Can you work these out from the drawing? Everything is in mm from the part's minimum corner. A direction names the side the tool comes from. Round coordinates to 2 decimals unless told otherwise and drop trailing zeros. Write each loop counter-clockwise with the first axis right and the second up, starting at its lowest first coordinate (ties: lowest second). Pieces come first, ordered by that corner, then holes. Notation, with made-up numbers: (-2, 53) -> (18, 53) arc R12 ccw to (18, 76) -> close; hole circle Ø2 at (42, 48). An arc over 180 degrees is marked (long way). Put each result on its own line as item: value. Start each with the question number.
1. Suppose I cut it at A-A (y = 6). Please give me the cut outline in (x, z).
2. For pin 1 (3 mm diameter, centred on x = 8, y = 10.5, fed in from +Z); pin 2 (1 mm diameter, centred on y = 4, z = 19, fed in from -X); pin 3 (2 mm diameter, centred on x = 18, z = 6.5, fed in from -Y); pin 4 (1.5 mm diameter, centred on x = 29.5, y = 8.5, fed in from +Z), each with a flat end and sliding along its axis, tell me the tip position at first contact or that it passes through.
3. Suppose I cut it at D-D (z = 19). Please give me the cut outline in (x, y).
4. Which directions (+Z, -Z, +X, -X, +Y, -Y) give clear straight access to the entire face, cutting with the end or side of a thin tool? Please do the marked faces 1, 2, 3, 4 and 5.
5. I need wall thicknesses on probe 1 along Y at (x, z) = (2.25, 16.85); probe 2 along Z at (x, y) = (20, 7.75); probe 3 along X at (y, z) = (7, 3.75). Which ranges of each line are inside material? Lowest first, please. Write a range as from..to.
6. Suppose I cut it at C-C (y = 8.5). Please give me the cut outline in (x, z).
7. Suppose I cut it at B-B (x = 2.25). Please give me the cut outline in (y, z), then the cut area to 3 significant figures.
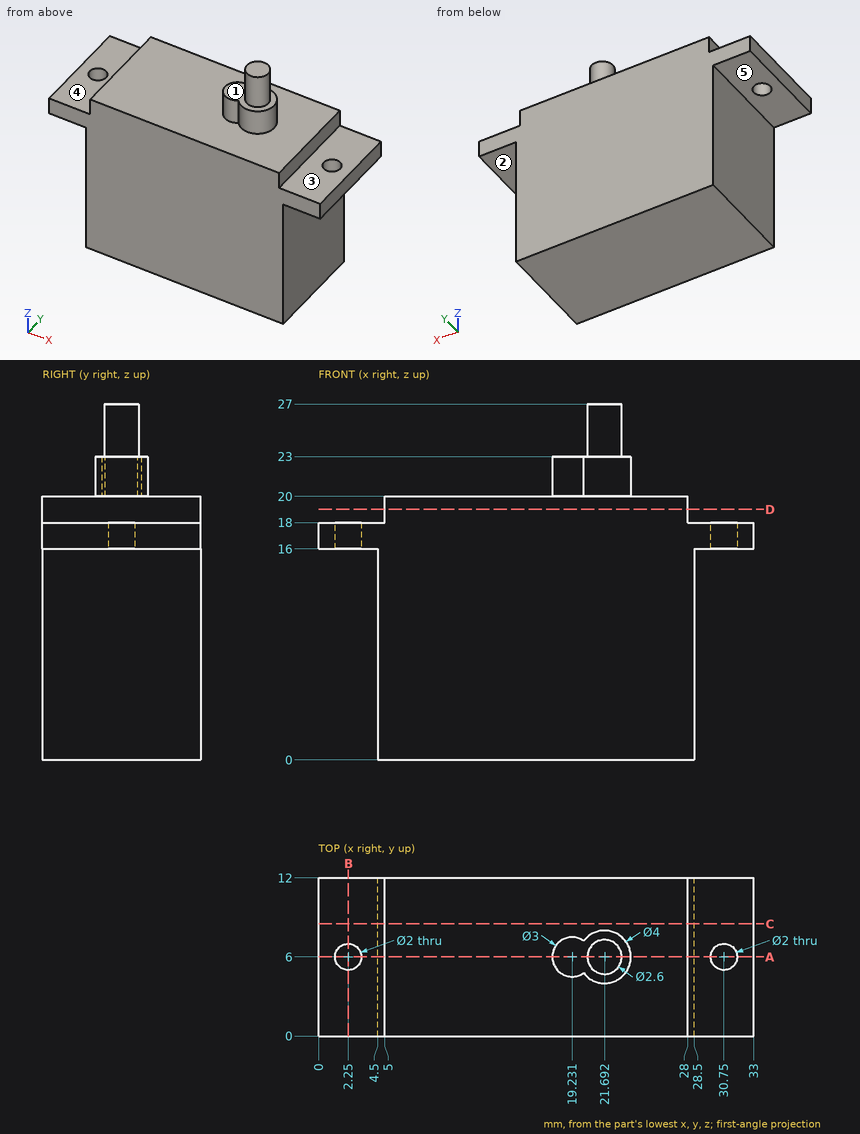
Verdict:
1. outline: (0, 16) -> (1.25, 16) -> (1.25, 18) -> (0, 18) -> close; (3.25, 16) -> (4.5, 16) -> (4.5, 0) -> (28.5, 0) -> (28.5, 16) -> (29.75, 16) -> (29.75, 18) -> (28, 18) -> (28, 20) -> (23.69, 20) -> (23.69, 23) -> (22.99, 23) -> (22.99, 27) -> (20.39, 27) -> (20.39, 23) -> (17.73, 23) -> (17.73, 20) -> (5, 20) -> (5, 18) -> (3.25, 18) -> close; (31.75, 16) -> (33, 16) -> (33, 18) -> (31.75, 18) -> close
2. pin 1: stops at z = 20
2. pin 2: stops at x = 5
2. pin 3: stops at y = 0
2. pin 4: stops at z = 18
3. outline: (5, 0) -> (28, 0) -> (28, 12) -> (5, 12) -> close
4. face 1: +Z
4. face 2: -Z, +X, +Y, -Y
4. face 3: +Z, +X, +Y, -Y
4. face 4: +Z, -X, +Y, -Y
4. face 5: -Z, -X, +Y, -Y
5. probe 1: y = 0..5, 7..12
5. probe 2: z = 0..20
5. probe 3: x = 4.5..28.5
6. outline: (0, 16) -> (4.5, 16) -> (4.5, 0) -> (28.5, 0) -> (28.5, 16) -> (33, 16) -> (33, 18) -> (28, 18) -> (28, 20) -> (5, 20) -> (5, 18) -> (0, 18) -> close
7. outline: (0, 16) -> (5, 16) -> (5, 18) -> (0, 18) -> close; (7, 16) -> (12, 16) -> (12, 18) -> (7, 18) -> close
7. area: 20.0 mm^2
